```python
from build123d import *

# Parameters (mm, degrees)
F1_DEPTH = 25
F3_DEPTH = 5
F4_DEPTH = 50
F5_R     = 5


with BuildPart() as f1:
    # F0 (on Top) → F1 (new body)
    with BuildSketch(Plane.XY):
        with BuildLine():
            Line((170, -160), (170, 3))
            Line((170, 3), (130, 43))
            Line((130, 43), (-20, 43))
            ThreePointArc((-20, 43), (-27.0710678119, 40.0710678119), (-30, 33))
            Line((-30, 33), (-30, -130))
            Line((-30, -130), (10, -170))
            Line((10, -170), (160, -170))
            ThreePointArc((160, -170), (167.0710678119, -167.0710678119), (170, -160))
        make_face()
        with BuildLine():
            ThreePointArc((24, -119.2476414861), (26.018165786, -113.2234965193), (31.2580645161, -109.630896205))
            ThreePointArc((31.2580645161, -109.630896205), (80.6101730553, -80.6101730553), (109.630896205, -31.2580645161))
            ThreePointArc((109.630896205, -31.2580645161), (113.2234965193, -26.018165786), (119.2476414861, -24))
            Line((119.2476414861, -24), (151, -24))
            ThreePointArc((151, -24), (158.0710678119, -26.9289321881), (161, -34))
            Line((161, -34), (161, -91))
            ThreePointArc((161, -91), (158.0710678119, -98.0710678119), (151, -101))
            Line((151, -101), (125, -101))
            ThreePointArc((125, -101), (108.0294372515, -108.0294372515), (101, -125))
            Line((101, -125), (101, -151))
            ThreePointArc((101, -151), (98.0710678119, -158.0710678119), (91, -161))
            Line((91, -161), (34, -161))
            ThreePointArc((34, -161), (26.9289321881, -158.0710678119), (24, -151))
            Line((24, -151), (24, -119.2476414861))
        make_face(mode=Mode.SUBTRACT)
        with BuildLine():
            ThreePointArc((53.8578643763, 14.1421356237), (82.1421356237, 14.1421356237), (82.1421356237, -14.1421356237))
            Line((82.1421356237, -14.1421356237), (14.1421356237, -82.1421356237))
            ThreePointArc((14.1421356237, -82.1421356237), (-14.1421356237, -82.1421356237), (-14.1421356237, -53.8578643763))
            Line((-14.1421356237, -53.8578643763), (53.8578643763, 14.1421356237))
        make_face(mode=Mode.SUBTRACT)
    extrude(amount=F1_DEPTH)

    # F2 (on face) → F3 (join)
    with BuildSketch(Plane(origin=(0, 0, 0), x_dir=(1, 0, 0), z_dir=(0, 0, -1))):
        with BuildLine():
            ThreePointArc((34, 161), (26.9289321881, 158.0710678119), (24, 151))
            Line((24, 151), (24, 119.2476414861))
            ThreePointArc((24, 119.2476414861), (26.018165786, 113.2234965193), (31.2580645161, 109.630896205))
            ThreePointArc((31.2580645161, 109.630896205), (80.6101730553, 80.6101730553), (109.630896205, 31.2580645161))
            ThreePointArc((109.630896205, 31.2580645161), (113.2234965193, 26.018165786), (119.2476414861, 24))
            Line((119.2476414861, 24), (151, 24))
            ThreePointArc((151, 24), (158.0710678119, 26.9289321881), (161, 34))
            Line((161, 34), (161, 91))
            ThreePointArc((161, 91), (158.0710678119, 98.0710678119), (151, 101))
            Line((151, 101), (125, 101))
            ThreePointArc((125, 101), (108.0294372515, 108.0294372515), (101, 125))
            Line((101, 125), (101, 151))
            ThreePointArc((101, 151), (98.0710678119, 158.0710678119), (91, 161))
            Line((91, 161), (34, 161))
        make_face()
    extrude(amount=-F3_DEPTH)

    # F2 (on face) → F4 (join)
    with BuildSketch(Plane(origin=(0, 0, 0), x_dir=(1, 0, 0), z_dir=(0, 0, -1))):
        with BuildLine():
            ThreePointArc((14.1421356237, 82.1421356237), (-14.1421356237, 82.1421356237), (-14.1421356237, 53.8578643763))
            Line((-14.1421356237, 53.8578643763), (53.8578643763, -14.1421356237))
            ThreePointArc((53.8578643763, -14.1421356237), (82.1421356237, -14.1421356237), (82.1421356237, 14.1421356237))
            Line((82.1421356237, 14.1421356237), (14.1421356237, 82.1421356237))
        make_face()
        with BuildLine():
            Line((60.9289321881, -7.0710678119), (-7.0710678119, 60.9289321881))
            ThreePointArc((-7.0710678119, 60.9289321881), (-7.0710678119, 75.0710678119), (7.0710678119, 75.0710678119))
            Line((7.0710678119, 75.0710678119), (75.0710678119, 7.0710678119))
            ThreePointArc((75.0710678119, 7.0710678119), (75.0710678119, -7.0710678119), (60.9289321881, -7.0710678119))
        make_face(mode=Mode.SUBTRACT)
    extrude(amount=-F4_DEPTH)

    # F5
    f5_edges = [f1.edges().sort_by_distance(p)[0] for p in [
        (19.857864, -19.857864, 25),
        (26.928932, -158.071068, 5),
        (24, -135.123821, 5),
        (26.018166, -113.223497, 5),
        (80.610173, -80.610173, 5),
        (113.223497, -26.018166, 5),
        (135.123821, -24, 5),
        (158.071068, -26.928932, 5),
        (161, -62.5, 5),
        (158.071068, -98.071068, 5),
        (138, -101, 5),
        (108.029437, -108.029437, 5),
        (101, -138, 5),
        (98.071068, -158.071068, 5),
        (62.5, -161, 5),
        (108.029437, -108.029437, 25),
    ]]
    fillet(f5_edges, radius=F5_R)


solid = f1.part
```
Geometry check sheet. Reference: the model listing, model coordinates, mm. A direction names the side the tool comes from. Coordinates: 2 decimals unless noted, no trailing zeros. Answer in a Markdown table with one row per item. Add a question column.
1. Gauge pin test, flat ends, axial feed: pin 1 Ø6 at (x, y) = (109.5, -65) entering from +Z; pin 2 Ø5 at (x, z) = (138, 13.5) entering from +Y; pin 3 Ø1 at (x, y) = (132, -8.5) entering from +Z. Record the tip position at first contact, or that the pin passes through.
2. Material ranges on L1, parallel to Z at x = 94, y = 34.5; L2, parallel to X at y = -33, z = 3.5; L3, parallel to X at y = -111, z = 8, recorded low to high. Write a range as [from, to].
3. Access from +Z, -Z, +X, -X, +Y, -Y to the whole of each face (thin tool, end or side, straight path). Record for faces 4 (the face through (-7.225, -74.914, 24.65)), 5 (the face through (138, -103, 24)).
4. Draft check along X on faces 1 (the face through (150, 23, 12)), 2 (the face through (135, -25, 7)), 3 (the face through (19.271, -18.319, 26.426)). Enter one of: +X half, -X half, draft (parallel to the pull), parting line (faces both ways), or undercut.
Data:
| question | item | result |
|---|---|---|
| 1 | pin 1 | stops at z = 5 |
| 1 | pin 2 | stops at y = 37.5 |
| 1 | pin 3 | stops at z = 25 |
| 2 | L1 | z = [0, 25] |
| 2 | L2 | x = [-30, 20.86], [49.14, 170] |
| 2 | L3 | x = [-30, 29.12], [104.99, 170] |
| 3 | face 4 | +Z, -Z |
| 3 | face 5 | +Z |
| 4 | face 1 | +X half |
| 4 | face 2 | undercut |
| 4 | face 3 | -X half |
